Check sheet for the drawn part. Datum: minimum x, y, z corner. Units: mm. Coordinates: 2 decimals unless noted, no trailing zeros. Loops run counter-clockwise (first coordinate to the right, second up) from the corner with the lowest first, then second, coordinate; pieces in that order, holes last. Notation, with made-up numbers: (71, -31.75) - (80, -31.75) arc R11 ccw to (80, -26.75) - close; hole circle Ø4 at (62, -20.5). An arc over 180 degrees is marked (long way). Answer as a JSON object with one key per item and string values. Group by question number.
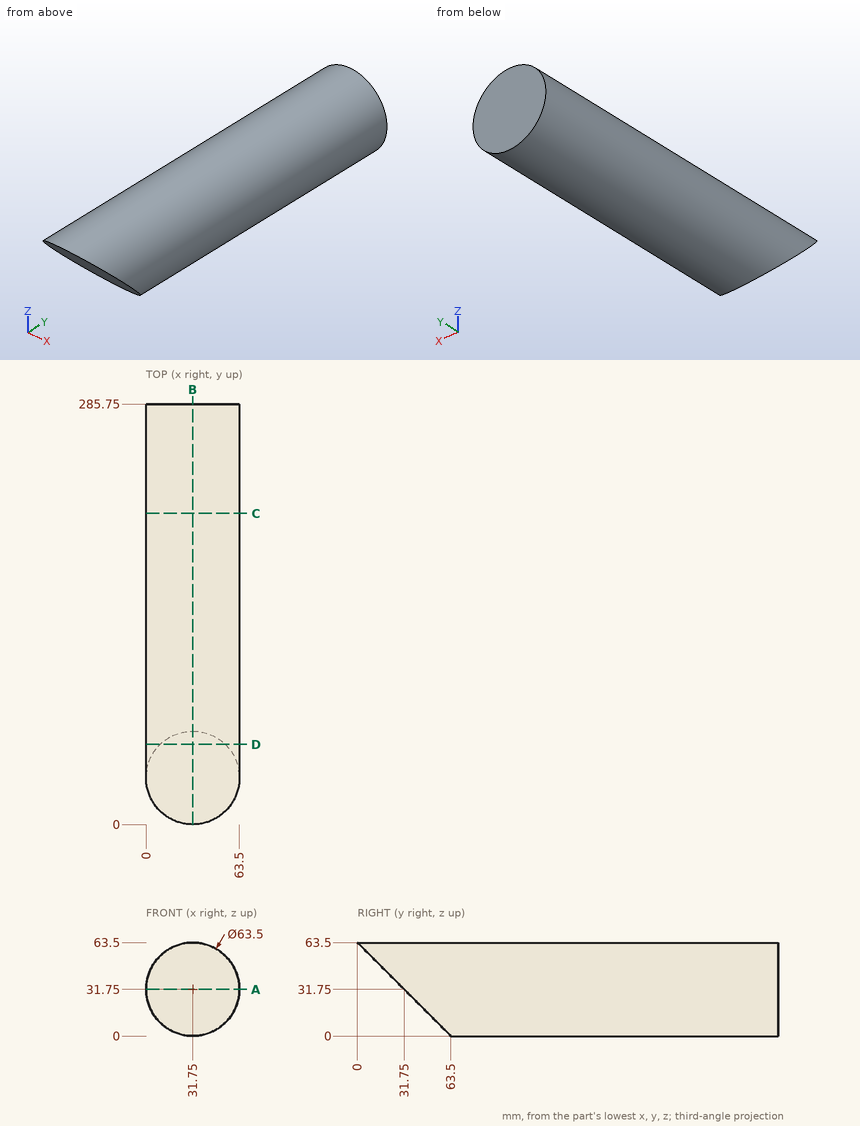
1. Sectioned sample at C-C on y = 211.5. Record the cut outline in (x, z).
2. Sectioned sample at D-D on y = 54.5. Record the cut outline in (x, z), plus the area to 3 significant figures.
3. Sectioned sample at A-A on z = 31.75. Record the cut outline in (x, y).
4. Sectioned sample at B-B on x = 31.75. Record the cut outline in (y, z), plus the area to 3 significant figures.
5. Material ranges on line 1 (X direction, y = 223.5, z = 32); line 2 (X direction, y = 81, z = 53.5); line 3 (Z direction, x = 52, y = 242), recorded low to high.
6. Gauge pin test, flat ends, axial feed: pin 1 (8 mm diameter, centred on x = 15.5, z = 17.5, fed in from -Y); pin 2 (3 mm diameter, centred on x = 13.5, y = 143, fed in from -Z); pin 3 (10 mm diameter, centred on x = 16, y = 200.5, fed in from +Z). Record the tip position at first contact, or that the pin passes through.
Answers follow:
{
 "1": {"outline": "circle Ø63.5 at (31.75, 31.75)"},
 "2": {"outline": "(9.6, 9) - (53.9, 9) arc R31.75 ccw (long way) to start", "area": "2,890 mm^2"},
 "3": {"outline": "(0, 31.75) - (63.5, 31.75) - (63.5, 285.75) - (0, 285.75) - close"},
 "4": {"outline": "(0, 63.5) - (63.5, 0) - (285.75, 0) - (285.75, 63.5) - close", "area": "16,100 mm^2"},
 "5": {"line 1": "x = 0 to 63.5", "line 2": "x = 8.62 to 54.88", "line 3": "z = 7.3 to 56.2"},
 "6": {"pin 1": "stops at y = 42", "pin 2": "stops at z = 4.78", "pin 3": "stops at z = 61.62"}
}
